from build123d import *

# Parameters (mm, degrees)
SKETCH1_R               = 57.15
SKETCH1_R_2             = 51.1302
EXTRUDE1_DEPTH          = 98.425
CUT_EXTRUDE1_DEPTH      = 128.356686613
CUT_EXTRUDE1_DEPTH_BACK = 128.356686613
CHAMFER4_SIZE           = 4.445
CHAMFER4_SIZE2          = 3.410768462


with BuildPart() as part:
    # Sketch1 → Extrude1 (new, symmetric)
    with BuildSketch(Plane.XY):
        Circle(SKETCH1_R)
        Circle(SKETCH1_R_2, mode=Mode.SUBTRACT)
    extrude(amount=EXTRUDE1_DEPTH, both=True)

    # Sketch4 → Cut-Extrude1 (cut, two sides: drawn at the far end of the back side and taken through both)
    with BuildSketch(Plane(origin=(0, 0, 0), x_dir=(1, 0, 0), z_dir=(0, 1, 0)).offset(-CUT_EXTRUDE1_DEPTH_BACK)):
        with BuildLine():
            Line((-57.15, -6.985), (-57.15, -98.425))
            Line((-57.15, -98.425), (57.15, -98.425))
            ThreePointArc((57.15, -98.425), (8.513587702, -42.063015372), (-57.15, -6.985))
        make_face()
    extrude(amount=CUT_EXTRUDE1_DEPTH + CUT_EXTRUDE1_DEPTH_BACK, mode=Mode.SUBTRACT)

    # Chamfer4
    chamfer4_edges = [part.edges().sort_by_distance(p)[0] for p in [
        (-57.15, 0, -98.425),
    ]]
    chamfer4_side = [part.faces().sort_by_distance(p)[0] for p in [
        (-55.533553898, 0, -98.425),
    ]]
    chamfer(chamfer4_edges, length=CHAMFER4_SIZE, length2=CHAMFER4_SIZE2, reference=chamfer4_side[0])


solid = part.part
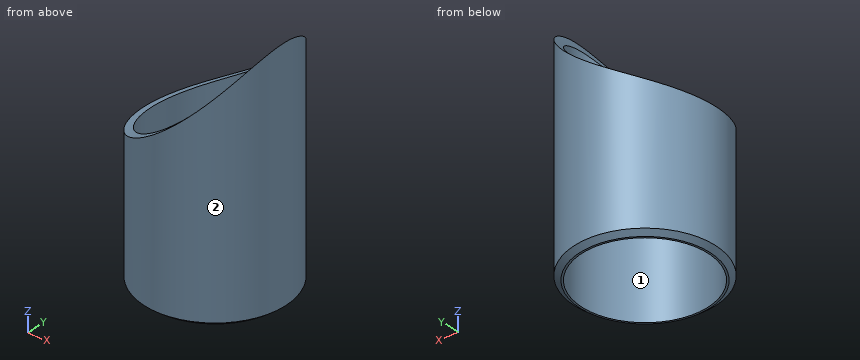
Design review of the part built by this model. Coordinates are the model's own, in mm. Face numbers are marked on the shaded views. Coordinates: 2 decimals unless noted, no trailing zeros. Loops run counter-clockwise (first coordinate to the right, second up) from the corner with the lowest first, then second, coordinate; pieces in that order, holes last. Notation, with made-up numbers: (20.5, -15) - (34.5, -15) arc R26 ccw to (34.5, 17) - close; hole circle Ø10 at (85.5, 32.25). An arc over 180 degrees is marked (long way). Use CSV: the item, a comma, the result in double quotes. Start each with the question number.
1. Mouldability with a two-part tool opening along Y and no side actions: class the marked faces 1 and 2 as released by +Y, released by -Y, zero draft, split by the parting line, or undercut.
2. Add section C-C on z = 47. Give the boundary of the cut face in (x, y), plus the area to 3 significant figures.
3. Clearance check with flat-ended pins moving along their axes: pin 1 (3 mm diameter, centred on y = 25.5, z = -7, fed in from +X); pin 2 (1 mm diameter, centred on x = 10, z = -34, fed in from +Y); pin 3 (1.5 mm diameter, centred on y = -3.5, z = -13, fed in from -X). State where each tip first meets the part, or that it passes through.
4. Add section A-A on x = 0. Give the boundary of the cut face in (y, z) (3 decimals).
5. To check wall thickness, follow probe 1 along Y at (x, z) = (0, 18); probe 2 along X at (y, z) = (0, 45). State the ranges of each line that lie inside material, in increasing order.
6. Add section B-B on z = -71.5. Give the boundary of the cut face in (x, y), plus the area to 3 significant figures.
Resolved:
1,face 1,"undercut"
1,face 2,"split by the parting line"
2,outline,"(14.45, -55.29) arc R57.15 ccw to (14.45, 55.29) - (14.45, 49.05) arc R51.13 cw to (14.45, -49.05) - close"
2,area,"848 mm2"
3,pin 1,"x = 51.87"
3,pin 2,"y = 56.35"
3,pin 3,"x = -57.08"
4,outline,"(-57.15, -95.014) - (-52.705, -98.425) - (-51.13, -98.425) - (-51.13, 35.611) - (-57.15, 35.611) - close; (51.13, -98.425) - (52.705, -98.425) - (57.15, -95.014) - (57.15, 35.611) - (51.13, 35.611) - close"
5,probe 1,"-57.15 to -51.13, 51.13 to 57.15"
5,probe 2,"51.13 to 57.15"
6,outline,"circle Ø114.3 at (0, 0); hole circle Ø102.26 at (0, 0)"
6,area,"2,050 mm2"
